Autodesk Inventor part; units mm, degrees
ref_plane "YZ Plane" through (0, 0, 0) normal (1, 0, 0) x (0, 1, 0)
ref_plane "XZ Plane" through (0, 0, 0) normal (0, 1, 0) x (-1, 0, 0)
ref_plane "XY Plane" through (0, 0, 0) normal (0, 0, 1) x (1, 0, 0)
sketch "Sketch1" plane through (0, 0, 0) normal (0, 1, 0) x (-1, 0, 0)
  circle A0 centre (0, 0) radius 200
  dimension "d0" = 400
extrude "Extrusion7" add sketch "Sketch1" along normal blind 3
ref_plane "Work Plane1" through (0, 3, 0) normal (0, 1, 0) x (1, 0, 0)
sketch "Sketch2" plane through (0, 3, 0) normal (0, 1, 0) x (1, 0, 0)
  line L0 (-63.5, -143.5) -> (63.5, -143.5)
  line L1 (63.5, -143.5) -> (63.5, 143.5)
  line L2 (63.5, 143.5) -> (-63.5, 143.5)
  line L3 (-63.5, 143.5) -> (-63.5, -143.5)
  line L4 (-63.5, -143.5) -> (63.5, 143.5) construction
  line L5 (63.5, -143.5) -> (-63.5, 143.5) construction
  point P0 (0, 0)
  dimension "d3" = 127
  dimension "d4" = 287
extrude "Extrusion2" cut sketch "Sketch2" against normal blind 3
ref_plane "Work Plane4" through (0, 3, 0) normal (0, 1, 0) x (1, 0, 0)
sketch "Sketch3" plane through (0, 3, 0) normal (0, 1, 0) x (1, 0, 0)
  line L0 (-63.5, 143.5) -> (-63.5, -143.5)
  line L1 (-63.5, 0) -> (-123.5, 0)
  line L2 (-123.5, 0) -> (-93.5, 0)
  line L3 (-93.5, 0) -> (-119.5, 0)
  circle A0 centre (-119.5, 0) radius 2.5
  circle A1 centre (-117.932, -8.8925) radius 2.5
  circle A2 centre (-113.4172, -16.7125) radius 2.5
  circle A3 centre (-106.5, -22.5167) radius 2.5
  circle A4 centre (-98.0149, -25.605) radius 2.5
  circle A5 centre (-88.9851, -25.605) radius 2.5
  circle A6 centre (-80.5, -22.5167) radius 2.5
  circle A7 centre (-73.5828, -16.7125) radius 2.5
  circle A8 centre (-69.068, -8.8925) radius 2.5
  circle A9 centre (-67.5, 0) radius 2.5
  circle A10 centre (-69.068, 8.8925) radius 2.5
  circle A11 centre (-73.5828, 16.7125) radius 2.5
  circle A12 centre (-80.5, 22.5167) radius 2.5
  circle A13 centre (-88.9851, 25.605) radius 2.5
  circle A14 centre (-98.0149, 25.605) radius 2.5
  circle A15 centre (-106.5, 22.5167) radius 2.5
  circle A16 centre (-113.4172, 16.7125) radius 2.5
  circle A17 centre (-117.932, 8.8925) radius 2.5
  line L4 (-93.5, 0) -> (-110.5, 0)
  line L5 (-110.5, 0) -> (-92.5712, 0)
  line L6 (-93.5, 0) -> (-103.5, 0)
  circle A18 centre (-110.5, 0) radius 2
  circle A19 centre (-103.5, 0) radius 1.5
  circle A20 centre (-109.4748, -5.8143) radius 2
  circle A21 centre (-106.5228, -10.9274) radius 2
  circle A22 centre (-102, -14.7224) radius 2
  circle A23 centre (-96.452, -16.7417) radius 2
  circle A24 centre (-90.548, -16.7417) radius 2
  circle A25 centre (-85, -14.7224) radius 2
  circle A26 centre (-80.4772, -10.9274) radius 2
  circle A27 centre (-77.5252, -5.8143) radius 2
  circle A28 centre (-76.5, 0) radius 2
  circle A29 centre (-77.5252, 5.8143) radius 2
  circle A30 centre (-80.4772, 10.9274) radius 2
  circle A31 centre (-85, 14.7224) radius 2
  circle A32 centre (-90.548, 16.7417) radius 2
  circle A33 centre (-96.452, 16.7417) radius 2
  circle A34 centre (-102, 14.7224) radius 2
  circle A35 centre (-106.5228, 10.9274) radius 2
  circle A36 centre (-109.4748, 5.8143) radius 2
  circle A37 centre (-101.5902, -5.8779) radius 1.5
  circle A38 centre (-96.5902, -9.5106) radius 1.5
  circle A39 centre (-90.4098, -9.5106) radius 1.5
  circle A40 centre (-85.4098, -5.8779) radius 1.5
  circle A41 centre (-83.5, 0) radius 1.5
  circle A42 centre (-85.4098, 5.8779) radius 1.5
  circle A43 centre (-90.4098, 9.5106) radius 1.5
  circle A44 centre (-96.5902, 9.5106) radius 1.5
  circle A45 centre (-101.5902, 5.8779) radius 1.5
  point P0 (0, 0)
  dimension "d7" = 60
  dimension "d8" = 30
  dimension "d9" = 26
  dimension "d10" = 5
  dimension "d13" = 360
  dimension "d15" = 17
  dimension "d16" = 10
  dimension "d18" = 4
  dimension "d19" = 3
  dimension "d22" = 360
  dimension "d26" = 360
extrude "Extrusion3" cut sketch "Sketch3" against normal blind 10
ref_plane "Work Plane2" through (0, 3, 0) normal (0, 1, 0) x (1, 0, 0)
sketch "Sketch4" plane through (0, 3, 0) normal (0, 1, 0) x (1, 0, 0)
  line L0 (0, 0) -> (0, -170)
  line L1 (0, -170) -> (0, 170)
  line L2 (0, -170) -> (-40, -170)
  line L3 (-40, -170) -> (-65, -170)
  line L4 (-65, -170) -> (0, -170)
  line L5 (0, -170) -> (65, -170)
  line L6 (0, 170) -> (-65, 170)
  line L7 (-65, 170) -> (0, 170)
  line L8 (0, 170) -> (65, 170)
  circle A0 centre (65, 170) radius 1.5
  circle A1 centre (-65, 170) radius 1.5
  circle A2 centre (-65, -170) radius 1.5
  circle A3 centre (65, -170) radius 1.5
  dimension "d30" = 170
  dimension "d31" = 340
  dimension "d32" = 40
  dimension "d33" = 25
  dimension "d34" = 65
  dimension "d35" = 65
  dimension "d36" = 65
  dimension "d37" = 65
  dimension "d38" = 65
  dimension "d39" = 3
  dimension "d40" = 3
  dimension "d41" = 3
  dimension "d42" = 3
extrude "Extrusion4" cut sketch "Sketch4" against normal blind 10
ref_plane "Work Plane3" through (0, 3, 0) normal (0, 1, 0) x (1, 0, 0)
properties part number "topplate" material "Birch"
Design review of the part built by this model. Coordinates are the model's own, in mm. Give positions to 0.01 mm unless a question says otherwise; leave off trailing zeros. Order: outer loops, then holes, each group sorted by start corner. A loop starts at its lowest first (then second) coordinate and runs counter-clockwise, first axis right, second up.
1. Add section A-A, the plane x = 0. State the section outline as (y, z) points, then the cut area to 3 significant figures.
Solution:
outline: (0, -200) - (3, -200) - (3, -143.5) - (0, -143.5) - close; (0, 143.5) - (3, 143.5) - (3, 200) - (0, 200) - close
area: 339 mm2
2. Add section D-D, the plane x = -144. State the section outline as (y, z) points.
Solution:
outline: (0, -138.79) - (3, -138.79) - (3, 138.79) - (0, 138.79) - close
3. For pin 1 Ø1 at (y, z) = (2.5, 78.5) entering from +X; pin 2 Ø1.5 at (y, z) = (1.5, -58) entering from +X; pin 3 Ø1 at (y, z) = (2.5, -133.5) entering from +X, all flat-tipped, find the tip position at first contact; note any pin that passes through.
Solution:
pin 1: stops at x = 184.16
pin 2: stops at x = 191.63
pin 3: stops at x = 149.37
4. Add section C-C, the plane y = 1.5. State how many separate pieces and enclosed holes the cut face has, then the cut area to 3 significant figures.
Solution:
separate pieces: 1
enclosed holes: 51
area: 88,500 mm2
5. To check wall thickness, follow L1, parallel to Z at x = 4, y = 0.4; L2, parallel to X at y = 1.05, z = 22; L3, parallel to Z at x = -113, y = 2.6. State the ranges of each line that lie inside material, in increasing order.
Solution:
L1: z = -199.96 to -143.5, 143.5 to 199.96
L2: x = -198.79 to -108.95, -104.05 to -82.95, -78.05 to -63.5, 63.5 to 198.79
L3: z = -165.02 to -19.18, -14.25 to 14.25, 19.18 to 165.02
6. Add section B-B, the plane z = -80. State the section outline as (x, y) points, then the cut area to 3 significant figures.
Solution:
outline: (-183.3, 0) - (-63.5, 0) - (-63.5, 3) - (-183.3, 3) - close; (63.5, 0) - (183.3, 0) - (183.3, 3) - (63.5, 3) - close
area: 719 mm2
